Source: CAD feature listing. Evaluate the final solid. Frame: model axes, mm. Round coordinates to 2 decimals unless told otherwise and drop trailing zeros. Loops run counter-clockwise (first coordinate to the right, second up) from the corner with the lowest first, then second, coordinate; pieces in that order, holes last.
Item 1: First-contact query: P1, Ø2, axis at x = 39.5, z = 7, coming from the +Y side; P2, Ø4, axis at x = 60.5, z = 4.5, coming from the -Y side; P3, Ø2, axis at y = -1.5, z = 2, coming from the -X side. Flat tips, straight axial feed; report the tip coordinate or a pass-through.
Item 2: Section query B-B on z = 2. Return loops of the section in (x, y).
Item 3: Ray query, L1, parallel to Y at x = 0, z = 7.75; L2, parallel to X at y = 1.75, z = 5; L3, parallel to X at y = -0.75, z = 8.25. Return the intervals inside material, ascending.
Item 4: Section query A-A on x = 26. Return loops of the section in (y, z), then the cut area to 3 significant figures.
```python
from build123d import *

# Parameters (mm, degrees)
SZKIC1_R                    = 5
SZKIC1_R_2                  = 4
DODANIE_WYCI_GNI_CIE1_DEPTH = 10
SZKIC2_W                    = 10
SZKIC2_H                    = 10
DODANIE_WYCI_GNI_CIE2_DEPTH = 10
DODANIE_WYCI_GNI_CIE3_DEPTH = 10
DODANIE_WYCI_GNI_CIE4_DEPTH = 10
SFAZOWANIE1_SIZE            = 10
DODANIE_WYCI_GNI_CIE6_START = 6
SZKIC6_R                    = 0.5
DODANIE_WYCI_GNI_CIE6_DEPTH = 210


with BuildPart() as part:
    # Szkic1 → Dodanie-wyci_gni_cie1 (new body)
    with BuildSketch(Plane.XY):
        Circle(SZKIC1_R)
        Circle(SZKIC1_R_2, mode=Mode.SUBTRACT)
    extrude(amount=DODANIE_WYCI_GNI_CIE1_DEPTH)



with BuildPart() as body_2:
    # Szkic2 → Dodanie-wyci_gni_cie2 (new body)
    with BuildSketch(Plane.XY.offset(10)):
        with Locations((10, 0)):
            Rectangle(SZKIC2_W, SZKIC2_H)
    extrude(amount=-DODANIE_WYCI_GNI_CIE2_DEPTH)


with BuildPart() as part_1:
    add(part.part)

    add(body_2.part)  # Dodanie-wyci_gni_cie3 merges body 2
    # Szkic3 → Dodanie-wyci_gni_cie3 (add)
    with BuildSketch(Plane.XY):
        Polygon((0, 5), (5, 5), (5, 0), (3.357304053, 3.705200331), align=None)
    extrude(amount=DODANIE_WYCI_GNI_CIE3_DEPTH)

    # Szkic5 → Dodanie-wyci_gni_cie4 (add)
    with BuildSketch(Plane(origin=(0, 0, 0), x_dir=(-1, 0, 0), z_dir=(0, 0, -1))):
        Polygon((-5, -5), (-5, 0), (-3.105231781, -3.918869172), (0, -5), align=None)
    extrude(amount=-DODANIE_WYCI_GNI_CIE4_DEPTH)

    # Sfazowanie1
    sfazowanie1_edges = [part_1.edges().sort_by_distance(p)[0] for p in [
        (15, 0, 10),
    ]]
    chamfer(sfazowanie1_edges, length=SFAZOWANIE1_SIZE - 0.0001)  # a hair under: the kernel refuses the full size

    # Szkic6 → Dodanie-wyci_gni_cie6 (add)
    with BuildSketch(Plane(origin=(0, 0, 0), x_dir=(0, 0, -1), z_dir=(1, 0, 0)).offset(DODANIE_WYCI_GNI_CIE6_START)):
        with Locations(Location((-5.785366317, 0, 0), (0, 0, 180))):
            Circle(SZKIC6_R)
    extrude(amount=DODANIE_WYCI_GNI_CIE6_DEPTH)


solid = part_1.part
```
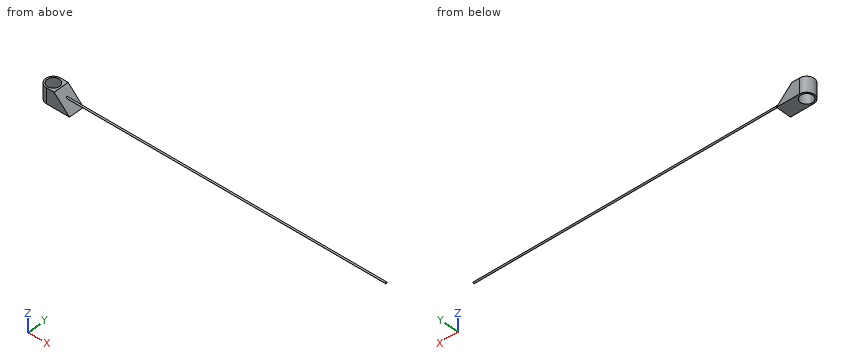
Data:
1. P1: stops at y = 0.45
1. P2: stops at y = -0.5
1. P3: stops at x = -4.97
2. outline: (0, -5) - (13, -5) - (13, 5) - (0, 5) arc R5 ccw to start; hole circle Ø8 at (0, 0)
3. L1: y = -5 to -4, 4 to 5
3. L2: x = -4.68 to -3.6, 3.6 to 10
3. L3: x = -4.94 to -3.93, 3.93 to 6.75
4. outline: circle Ø1 at (0, 5.79)
4. area: 0.785 mm2
